Read the model definition and answer for the solid it produces. Units are mm, in the model's axes. Face numbers are marked on the shaded views. A direction names the side the tool comes from. Give positions to 0.01 mm unless a question says otherwise; leave off trailing zeros. Order: outer loops, then holes, each group sorted by start corner. A loop starts at its lowest first (then second) coordinate and runs counter-clockwise, first axis right, second up. Notation, with made-up numbers: (17, 53.25) - (30, 53.25) arc R19 cw to (30, 64.25) - close; hole circle Ø1 at (30, -25.5). An arc over 180 degrees is marked (long way). Write item = value, one per line.
```python
from build123d import *

# Parameters (mm, degrees)
F1_DEPTH = 6.35
F2_DEPTH = 53.848
F3_DEPTH = 12.7
F5_R     = 3.81
F6_DEPTH = 51.116
F7_R     = 1.27
F8_R     = 1.27


with BuildPart() as f1:
    # F0 (on Front) → F1 (new body)
    with BuildSketch(Plane.XZ):
        with BuildLine():
            Line((-20, 20), (0, 0))
            Line((0, 0), (20, 20))
            Line((20, 20), (5.715, 20))
            ThreePointArc((5.715, 20), (0, 14.285), (-5.715, 20))
            Line((-5.715, 20), (-20, 20))
        make_face()
    extrude(amount=F1_DEPTH)

    # F0 (on Front) → F2 (join)
    with BuildSketch(Plane.XZ):
        with BuildLine():
            ThreePointArc((-5.715, 20), (0, 14.285), (5.715, 20))
            Line((5.715, 20), (-5.715, 20))
        make_face()
        with BuildLine():
            Line((-5.715, 20), (5.715, 20))
            ThreePointArc((5.715, 20), (0, 25.715), (-5.715, 20))
        make_face()
    extrude(amount=F2_DEPTH)

    # F0 (on Front) → F3 (join)
    with BuildSketch(Plane.XZ):
        with BuildLine():
            ThreePointArc((-5.715, 20), (0, 25.715), (5.715, 20))
            Line((5.715, 20), (5.715, 45.4))
            Line((5.715, 45.4), (-5.715, 45.4))
            Line((-5.715, 45.4), (-5.715, 20))
        make_face()
    extrude(amount=F3_DEPTH)

    # F5 (on offset) → F6 (cut, through all)
    with BuildSketch(Plane.YZ.offset(31.115)):
        with Locations((-6.35, 35.24)):
            Circle(F5_R)
    extrude(amount=-F6_DEPTH, mode=Mode.SUBTRACT)

    # F7
    f7_edges = [f1.edges().sort_by_distance(p)[0] for p in [
        (5.715, -10.16, 35.24),
        (-5.715, -10.16, 35.24),
    ]]
    fillet(f7_edges, radius=F7_R)

    # F8
    f8_edges = [f1.edges().sort_by_distance(p)[0] for p in [
        (-20, -3.175, 20),
        (20, -3.175, 20),
    ]]
    fillet(f8_edges, radius=F8_R)


solid = f1.part
```
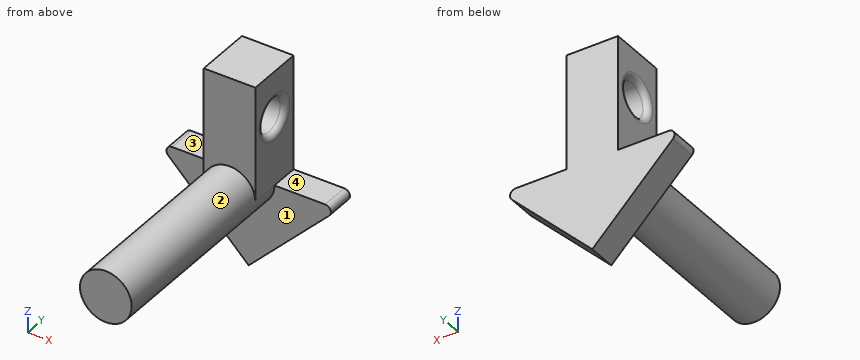
1. Section B-B (x = -8) is taken. Determine the outline of the cut face in (y, z), and give its area (3 significant figures).
Recorded:
outline = (-6.35, 8) - (0, 8) - (0, 20) - (-6.35, 20) - close
area = 76.2 mm^2
2. Section D-D (z = 29.5) is taken. Determine the outline of the cut face in (x, y) (3 decimals), and give its area (3 significant figures).
Recorded:
outline = (-5.715, -12.7) - (5.715, -12.7) - (5.715, 0) - (-5.715, 0) - close
area = 145 mm^2
3. Flat-ended cylindrical pins translate along their axes: pin 1 (12 mm diameter, centred on y = -6.35, z = 35.24, fed in from -X) (3 decimals); pin 2 (1.5 mm diameter, centred on x = -2.5, y = -29, fed in from +Z); pin 3 (5 mm diameter, centred on y = -29, z = 24, fed in from -X); pin 4 (16 mm diameter, centred on x = -7.5, z = 11.5, fed in from -Y). Find the tip coordinate at first contact, or state that the pin passes through.
Recorded:
pin_1 = -5.715
pin_2 = 25.44
pin_3 = -5.51
pin_4 = -53.85
4. Section A-A (z = 35.24) is taken. Determine the outline of the cut face in (x, y) (3 decimals).
Recorded:
outline = (-5.715, -12.7) - (5.715, -12.7) - (5.715, -11.43) arc R1.27 ccw to (4.445, -10.16) - (-4.445, -10.16) arc R1.27 ccw to (-5.715, -11.43) - close; (-5.715, -1.27) arc R1.27 ccw to (-4.445, -2.54) - (4.445, -2.54) arc R1.27 ccw to (5.715, -1.27) - (5.715, 0) - (-5.715, 0) - close
5. Straight lines are drawn through the part: L1, parallel to Y at x = 2, z = 35; L2, parallel to Y at x = 3, z = 42; L3, parallel to Y at x = -3.5, z = 11. For each, find the intervals that lie inside material, in ascending order. Write a range as [from, to].
Recorded:
L1 = [-12.7, -10.15], [-2.55, 0]
L2 = [-12.7, 0]
L3 = [-6.35, 0]
6. Section C-C (y = -23) is taken. Determine the outline of the cut face in (x, z) (3 decimals).
Recorded:
outline = circle Ø11.43 at (0, 20)
7. For the marked faces 1, 2, 3 and 4, determine the directions among +Z, -Z, +X, -X, +Y, -Y from which every point of the face is accessible in a straight line to the end or side of a thin tool.
Recorded:
face_1 = -Z, -Y
face_2 = -Y
face_3 = +Z, -X, +Y, -Y
face_4 = +Z, +X, +Y, -Y
